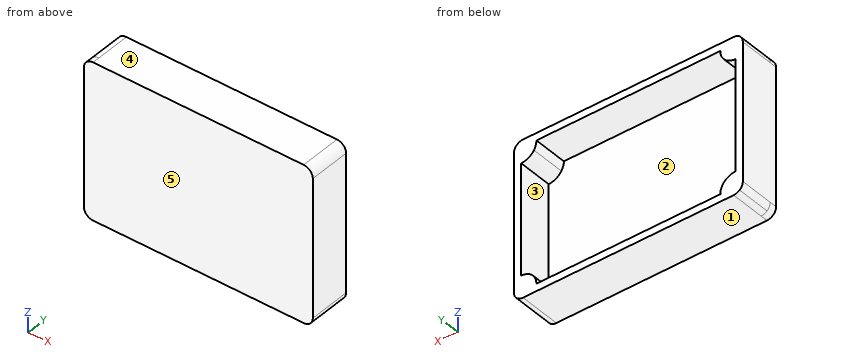
from build123d import *

# Parameters (mm, degrees)
BOSS_EXTRUDE1_DEPTH = 3.2
BOSS_EXTRUDE2_DEPTH = 15


with BuildPart() as part:
    # Sketch1 → Boss-Extrude1 (new body)
    with BuildSketch(Plane(origin=(0, 0, 0), x_dir=(1, 0, 0), z_dir=(0, 1, 0))):
        with BuildLine():
            Line((-46, -34), (46, -34))
            ThreePointArc((46, -34), (48.828427125, -32.828427125), (50, -30))
            Line((50, -30), (50, 30))
            ThreePointArc((50, 30), (48.828427125, 32.828427125), (46, 34))
            Line((46, 34), (-46, 34))
            ThreePointArc((-46, 34), (-48.828427125, 32.828427125), (-50, 30))
            Line((-50, 30), (-50, -30))
            ThreePointArc((-50, -30), (-48.828427125, -32.828427125), (-46, -34))
        make_face()
    extrude(amount=BOSS_EXTRUDE1_DEPTH)

    # Sketch2 → Boss-Extrude2 (add)
    with BuildSketch(Plane(origin=(0, 3.2, 0), x_dir=(1, 0, 0), z_dir=(0, 1, 0))):
        with BuildLine():
            ThreePointArc((-48.594612634, -33.044336591), (-47.382507439, -33.753488135), (-46, -34))
            Line((-46, -34), (46, -34))
            ThreePointArc((46, -34), (48.828427125, -32.828427125), (50, -30))
            Line((50, -30), (50, 30))
            ThreePointArc((50, 30), (48.828427125, 32.828427125), (46, 34))
            Line((46, 34), (-46, 34))
            ThreePointArc((-46, 34), (-47.382507439, 33.753488135), (-48.594612634, 33.044336591))
            ThreePointArc((-48.594612634, 33.044336591), (-49.631697298, 31.676536529), (-50, 30))
            Line((-50, 30), (-50, -27.196030412))
            Line((-50, -27.196030412), (-50, -30))
            ThreePointArc((-50, -30), (-49.631697298, -31.676536529), (-48.594612634, -33.044336591))
        make_face()
        with BuildLine():
            ThreePointArc((-41.245050157, -27.144178308), (-43.644743612, -24.94621002), (-46.8, -24.15))
            Line((-46.8, -24.15), (-46.8, 24.15))
            ThreePointArc((-46.8, 24.15), (-43.644743612, 24.94621002), (-41.245050157, 27.144178308))
            ThreePointArc((-41.245050157, 27.144178308), (-40.429642221, 28.891848598), (-40.15, 30.8))
            Line((-40.15, 30.8), (40.166928077, 30.8))
            ThreePointArc((40.166928077, 30.8), (40.445858448, 28.896705942), (41.259190701, 27.153484478))
            ThreePointArc((41.259190701, 27.153484478), (43.652775555, 24.961111285), (46.8, 24.166928077))
            Line((46.8, 24.166928077), (46.8, -24.15))
            ThreePointArc((46.8, -24.15), (43.644743612, -24.94621002), (41.245050157, -27.144178308))
            ThreePointArc((41.245050157, -27.144178308), (40.429642221, -28.891848598), (40.15, -30.8))
            Line((40.15, -30.8), (-40.15, -30.8))
            ThreePointArc((-40.15, -30.8), (-40.429642221, -28.891848598), (-41.245050157, -27.144178308))
        make_face(mode=Mode.SUBTRACT)
    extrude(amount=BOSS_EXTRUDE2_DEPTH)


solid = part.part
Check sheet for the modelled part. Datum: model origin and axes. Units: mm. Face numbers are marked on the shaded views. A direction names the side the tool comes from. Give positions to 0.01 mm unless a question says otherwise; leave off trailing zeros. Order: outer loops, then holes, each group sorted by start corner. A loop starts at its lowest first (then second) coordinate and runs counter-clockwise, first axis right, second up. Notation, with made-up numbers: (60.5, -35.5) - (109.5, -35.5) arc R28 ccw to (109.5, -8.5) - close; hole circle Ø5 at (-32.5, 29.5). An arc over 180 degrees is marked (long way). Answer as CSV lines item,"result".
1. Section check C-C (x = 25.5). Record the boundary of the cut face in (y, z).
Result sheet:
outline,"(0, -34) - (18.2, -34) - (18.2, -30.8) - (3.2, -30.8) - (3.2, 30.8) - (18.2, 30.8) - (18.2, 34) - (0, 34) - close"
2. Go/stop test with a flat-tipped pin: P1, Ø5, axis at x = 19, z = 11, coming from the +Y side. Record where the tip stops, or that it passes through.
Result sheet:
P1,"y = 3.2"
3. Tool access check on the marked faces 1 and 2. Record the directions out of +Z, -Z, +X, -X, +Y, -Y that give a thin tool (end or side, any length) a straight path to the whole face; none if there is none.
Result sheet:
face 1,"-Z, +X, -X, +Y, -Y"
face 2,"+Y"
4. Section check B-B (z = 13.5). Record the boundary of the cut face in (x, y).
Result sheet:
outline,"(-50, 0) - (50, 0) - (50, 18.2) - (46.8, 18.2) - (46.8, 3.2) - (-46.8, 3.2) - (-46.8, 18.2) - (-50, 18.2) - close"
5. Scan lines: probe 1 along Z at (x, y) = (23, 3.5); probe 2 along X at (y, z) = (10.5, -19.5); probe 3 along Y at (x, z) = (-13, 12.5). Record each from-to range of solid material in increasing order. Write a range as from..to.
Result sheet:
probe 1,"-34..-30.8, 30.8..34"
probe 2,"-50..-46.8, 46.8..50"
probe 3,"0..3.2"
6. Section check A-A (y = 10.25). Record the boundary of the cut face in (x, z), then the cut area to 3 significant figures.
Result sheet:
outline,"(-50, -30) arc R4 ccw to (-46, -34) - (46, -34) arc R4 ccw to (50, -30) - (50, 30) arc R4 ccw to (46, 34) - (-46, 34) arc R4 ccw to (-50, 30) - close; hole (-46.8, -24.15) arc R6.65 cw to (-40.15, -30.8) - (40.17, -30.8) arc R6.63 cw to (46.8, -24.17) - (46.8, 24.15) arc R6.65 cw to (40.15, 30.8) - (-40.15, 30.8) arc R6.65 cw to (-46.8, 24.15) - close"
area,"1,160 mm²"
7. Mould release check, pull along Z, two halves, no side actions. Record for the marked faces 3, 4 and 5: released by +Z, released by -Z, zero draft, split by the parting line, or undercut.
Result sheet:
face 3,"undercut"
face 4,"released by +Z"
face 5,"zero draft"
